from build123d import *

# Parameters (mm, degrees)
SKETCH1_W                        = 40
SKETCH1_H                        = 20
SKETCH1_R                        = 2.38
BOSS_EXTRUDE1_DEPTH              = 25
F_11_64_0_17188_DIAMETER_HOLE1_D = 4.365752


with BuildPart() as part:
    # Sketch1 → Boss-Extrude1 (new body)
    with BuildSketch(Plane(origin=(0, 0, 0), x_dir=(1, 0, 0), z_dir=(0, 1, 0))):
        with Locations((20, 10)):
            Rectangle(SKETCH1_W, SKETCH1_H)
        with Locations(Location((10, 14, 0), (0, 0, 270))):  # turned: the seam where the file's is
            Circle(SKETCH1_R, mode=Mode.SUBTRACT)
        with Locations(Location((30, 14, 0), (0, 0, 270))):  # turned: the seam where the file's is
            Circle(SKETCH1_R, mode=Mode.SUBTRACT)
    extrude(amount=BOSS_EXTRUDE1_DEPTH)

    # 11/64 (0.17188) Diameter Hole1 (through all)
    with Locations(Plane(origin=(0, 25, 0), x_dir=(1, 0, 0), z_dir=(0, 1, 0))):
        with Locations((20, 14)):
            Hole(F_11_64_0_17188_DIAMETER_HOLE1_D / 2)


solid = part.part
Part model, mm, in its own coordinate system. Give positions to 0.01 mm unless a question says otherwise; leave off trailing zeros. Write each loop counter-clockwise with the first axis right and the second up, starting at its lowest first coordinate (ties: lowest second). Pieces come first, ordered by that corner, then holes.
1) Pin check, flat tip, straight feed: pin 1 (3 mm diameter, centred on x = 30, z = -14, fed in from -Y). Stop position of the tip, or through.
Resolved:
pin 1: passes through
2) Cut at A-A on x = 20. Write the cut outline in (y, z).
Resolved:
outline: (0, -20) - (25, -20) - (25, -16.18) - (0, -16.18) - close; (0, -11.82) - (25, -11.82) - (25, 0) - (0, 0) - close
3) Cut at B-B on z = -14. Write the cut outline in (x, y).
Resolved:
outline: (0, 0) - (7.62, 0) - (7.62, 25) - (0, 25) - close; (12.38, 0) - (17.82, 0) - (17.82, 25) - (12.38, 25) - close; (22.18, 0) - (27.62, 0) - (27.62, 25) - (22.18, 25) - close; (32.38, 0) - (40, 0) - (40, 25) - (32.38, 25) - close
4) Cut at C-C on y = 17.5. Write the cut outline in (x, z).
Resolved:
outline: (0, -20) - (40, -20) - (40, 0) - (0, 0) - close; hole circle Ø4.76 at (10, -14); hole circle Ø4.37 at (20, -14); hole circle Ø4.76 at (30, -14)
5) Two-plate mould, pull along Z, no slides. Class faces 1 (the face through (20, 12, -20)), 2 (the face through (20, 0, -10)), 3 (the face through (27.677, 12.325, -14.516)): released by +Z, released by -Z, zero draft, split by the parting line, or undercut.
Resolved:
face 1: released by -Z
face 2: zero draft
face 3: undercut
6) Probe L1, parallel to X at y = 6.5, z = -14; L2, parallel to Z at x = 20, y = 6.75; L3, parallel to Z at x = 22, y = 16. List the from-to ranges inside material, lowest first.
Resolved:
L1: x = 0 to 7.62, 12.38 to 17.82, 22.18 to 27.62, 32.38 to 40
L2: z = -20 to -16.18, -11.82 to 0
L3: z = -20 to -14.87, -13.13 to 0
7) Cut at D-D on x = 10. Write the cut outline in (y, z).
Resolved:
outline: (0, -20) - (25, -20) - (25, -16.38) - (0, -16.38) - close; (0, -11.62) - (25, -11.62) - (25, 0) - (0, 0) - close
